Here's how the part is built. I have some questions about the finished solid (model axes, mm). A direction names the side the tool comes from. Round coordinates to 2 decimals unless told otherwise and drop trailing zeros. Loops run counter-clockwise (first coordinate to the right, second up) from the corner with the lowest first, then second, coordinate; pieces in that order, holes last. Notation, with made-up numbers: (20.5, -23) - (69.5, -23) arc R35 ccw to (69.5, 14) - close; hole circle Ø3 at (-32.75, 12). An arc over 180 degrees is marked (long way). Return JSON: item names as keys, results as strings. Group by question number.
```python
from build123d import *

# Parameters (mm, degrees)
BASE_FLANGE1_DEPTH      = 11
FILLET1_R               = 10
CUT_EXTRUDE1_DEPTH      = 190.414888538
CUT_EXTRUDE1_DEPTH_BACK = 190.414888538
SKETCH7_R               = 5.894184215
BODY_MOVE_COPY1_ANGLE   = 120


# Sheet-metal steps are written as plain solids
with BuildPart() as part:
    # Sketch2 → Base-Flange1 (new, symmetric)
    with BuildSketch(Plane.XY):
        with BuildLine():
            Line((-189, 0), (-0.1, 0))
            ThreePointArc((-0.1, 0), (-0.029289322, 0.029289322), (0, 0.1))
            Line((0, 0.1), (0, 3.9))
            ThreePointArc((0, 3.9), (0.61507576, 5.38492424), (2.1, 6))
            Line((2.1, 6), (32, 6))
            Line((32, 6), (32, 4))
            Line((32, 4), (2.1, 4))
            ThreePointArc((2.1, 4), (2.029289322, 3.970710678), (2, 3.9))
            Line((2, 3.9), (2, 0.1))
            ThreePointArc((2, 0.1), (1.38492424, -1.38492424), (-0.1, -2))
            Line((-0.1, -2), (-189, -2))
            Line((-189, -2), (-189, 0))
        make_face()
    extrude(amount=BASE_FLANGE1_DEPTH, both=True)

    # Fillet1
    fillet1_edges = [part.edges().sort_by_distance(p)[0] for p in [
        (-189, -1, -11),
        (32, 5, -11),
        (-189, -1, 11),
        (32, 5, 11),
    ]]
    fillet(fillet1_edges, radius=FILLET1_R)

    # Sketch7 → Cut-Extrude1 (cut, two sides: drawn at the far end of the back side and taken through both)
    with BuildSketch(Plane(origin=(0, 0, 0), x_dir=(1, 0, 0), z_dir=(0, 1, 0)).offset(-CUT_EXTRUDE1_DEPTH_BACK)):
        with Locations(Location((-179, 0, 0), (0, 0, 270))):
            Circle(SKETCH7_R)
        with BuildLine():
            Line((20.46881318, 0.616566496), (23.297240305, 0.616566496))
            ThreePointArc((23.297240305, 0.616566496), (21.883026743, -1.383433504), (20.46881318, 0.616566496))
        make_face()
    extrude(amount=CUT_EXTRUDE1_DEPTH + CUT_EXTRUDE1_DEPTH_BACK, mode=Mode.SUBTRACT)


with BuildPart() as part_1:
    # Body-Move/Copy1: moved
    add(part.part.moved(Location((0, 0, 0))).rotate(Axis((-95.951666667, -47.903333333, 48.048333333), (-0.5773502691898587, 0.5773502691889744, -0.5773502691900443)), BODY_MOVE_COPY1_ANGLE))


solid = part_1.part
```
Q1. Imagine slicing it at D-D, the plane z = -2.5. List the corners of the cut face in (x, y) for me (3 decimals).
Q2. Imagine slicing it at C-C, the plane x = -152.75. List the corners of the cut face in (y, z) for me (3 decimals), and give its area (3 significant figures).
Q3. Imagine slicing it at B-B, the plane y = -128. List the corners of the cut face in (x, z) for me (3 decimals).
Q4. Please list where these lines run through material, in increasing order: line 1 (Y direction, x = -153.5, z = -3.25) (3 decimals); line 2 (Z direction, x = -134.25, y = -26) (3 decimals); line 3 (Y direction, x = -144, z = 0.7) (3 decimals).
Q5. Will these pins go through, and if not, where does the flat tip stop? pin 1 Ø3 at (x, z) = (-136, -4.5) entering from -Y; pin 2 Ø3.5 at (x, y) = (-144.12, -165.74) entering from -Z (3 decimals); pin 3 Ø3 at (x, y) = (-139.5, -63) entering from -Z (3 decimals); pin 4 Ø6.5 at (x, y) = (-140, -156.5) entering from +Z (3 decimals).
Q6. Imagine slicing it at A-A, the plane x = -140.5. List the corners of the cut face in (y, z) for me (3 decimals).
Q7. If we mould it in two halves opening along X, with no side actions, what happens to faces 4 (the flat face through (-155, -66, 1)), 5 (the cylindrical face through (-135.852, 42.138, 1.131)), 6 (the flat face through (-144, -145.855, -2)), 7 (the cylindrical face through (-138.555, 37.403, 1.159))? For each: +X half, -X half, draft (parallel to the pull), parting line (faces both ways), or undercut.
Q8. For faces 1 (the flat face through (-144, -143.855, -2)), 2 (the flat face through (-144, -161, -3.855)), 3 (the flat face through (-144, -51, 2.145)), which set-ups out of +Z, -Z, +X, -X, +Y, -Y let a thin tool reach every point of the face, with its end or its side?
Output values:
{
 "1": {"outline": "(-155, -145.855) - (-133, -145.855) - (-133, -143.855) - (-155, -143.855) - close"},
 "2": {"outline": "(-172.175, -5.855) - (-145.955, -5.855) arc R2.1 ccw to (-143.855, -3.755) - (-143.855, 0.045) arc R0.1 cw to (-143.755, 0.145) - (41.465, 0.145) - (41.465, 2.145) - (-143.755, 2.145) arc R2.1 ccw to (-145.855, 0.045) - (-145.855, -3.755) arc R0.1 cw to (-145.955, -3.855) - (-172.175, -3.855) - close", "area": "437 mm^2"},
 "3": {"outline": "(-155, 0.145) - (-133, 0.145) - (-133, 2.145) - (-155, 2.145) - close"},
 "4": {"line 1": "y = -145.855 to -143.855", "line 2": "z = 0.145 to 2.145", "line 3": "y = -145.75 to 29.251, 41.039 to 45.145"},
 "5": {"pin 1": "stops at y = -174.21", "pin 2": "stops at z = -5.855", "pin 3": "stops at z = 0.145", "pin 4": "stops at z = -3.855"},
 "6": {"outline": "(-175.537, -5.855) - (-145.955, -5.855) arc R2.1 ccw to (-143.855, -3.755) - (-143.855, 0.045) arc R0.1 cw to (-143.755, 0.145) - (30.402, 0.145) - (30.402, 2.145) - (-143.755, 2.145) arc R2.1 ccw to (-145.855, 0.045) - (-145.855, -3.755) arc R0.1 cw to (-145.955, -3.855) - (-175.537, -3.855) - close; (39.888, 0.145) - (44.827, 0.145) - (44.827, 2.145) - (39.888, 2.145) - close"},
 "7": {"face 4": "-X half", "face 5": "+X half", "face 6": "draft", "face 7": "undercut"},
 "8": {"face 1": "-Z, +X, -X, +Y", "face 2": "+Z, +X, -X, -Y", "face 3": "+Z, +X, -X, +Y, -Y"}
}
